Here's the drawing with two shaded views (mm, measured from the low corner). I have some questions. A direction names the side the tool comes from. Round coordinates to 2 decimals unless told otherwise and drop trailing zeros. Order: outer loops, then holes, each group sorted by start corner. A loop starts at its lowest first (then second) coordinate and runs counter-clockwise, first axis right, second up.
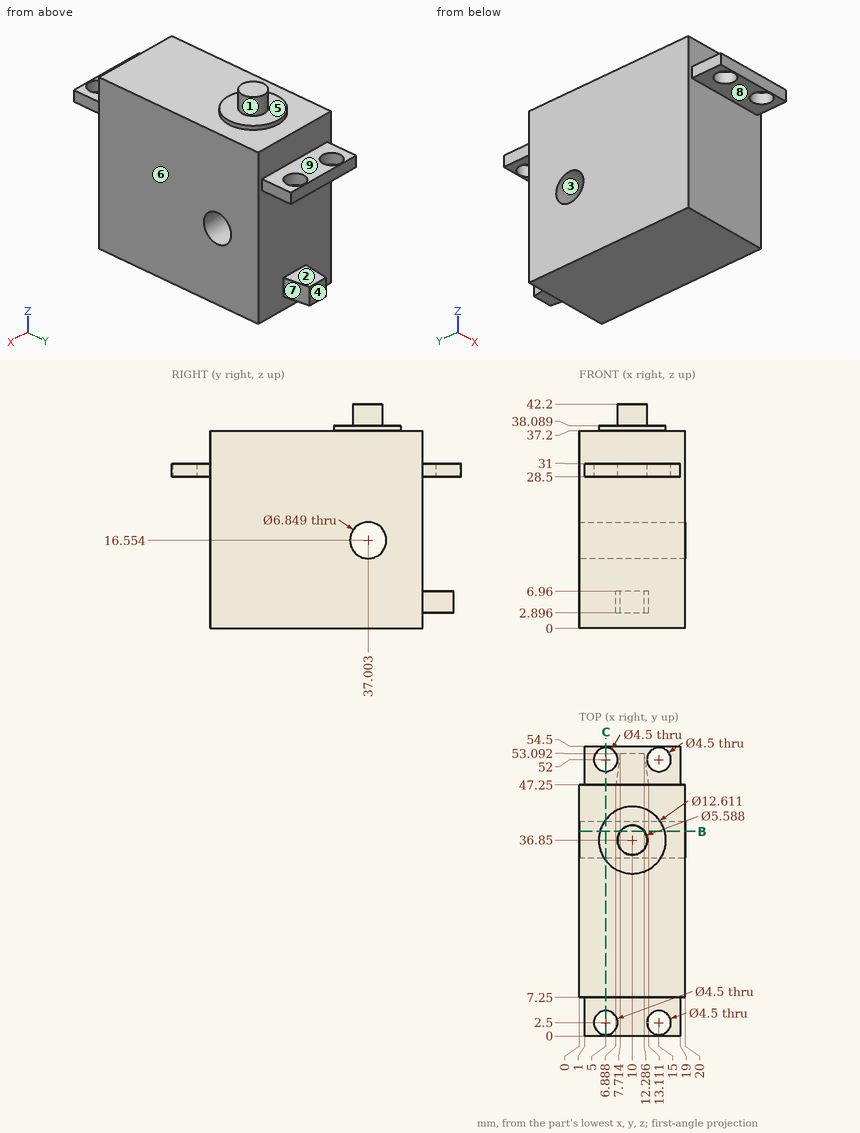
Q1. I need wall thicknesses on L1, parallel to Y at x = 5, z = 29; L2, parallel to Z at x = 16, y = 48.5; L3, parallel to Z at x = 15, y = 18.5. Which ranges of each line are inside material? Lowest first, please.
Q2. We'd pull the mould along Y, two halves only. Please class the marked faces 1, 2, 3 and 4: released by +Y, released by -Y, zero draft, split by the parting line, or undercut.
Q3. For P1, Ø1.5, axis at x = 6, z = 7, coming from the +Y side; P2, Ø6, axis at x = 5, y = 52, coming from the +Z side; P3, Ø6, axis at x = 14, z = 4, coming from the +Y side; P4, Ø5, axis at y = 28.5, z = 20, coming from the -X side, each with a flat end and sliding along its axis, tell me the tip position at first contact or that it passes through.
Q4. Imagine slicing it at B-B, the plane y = 38.5. Please give me the cut outline in (x, z) (1 decimal).
Q5. For the marked faces 5, 6, 7, 8 and 9, which set-ups out of +Z, -Z, +X, -X, +Y, -Y let a thin tool reach every point of the face, with its end or its side?
Q6. Imagine slicing it at C-C, the plane x = 5. State how many separate pieces and enclosed holes the cut face has, then the cut area to 3 significant figures.
Filled in:
1. L1: y = 0 to 0.25, 4.75 to 49.75, 54.25 to 54.5
1. L2: z = 28.5 to 31
1. L3: z = 0 to 37.2
2. face 1: split by the parting line
2. face 2: zero draft
2. face 3: undercut
2. face 4: released by +Y
3. P1: stops at y = 47.25
3. P2: stops at z = 31
3. P3: stops at y = 53.09
3. P4: stops at x = 0
4. outline: (0, 0) - (20, 0) - (20, 13.5) - (0, 13.5) - close; (0, 19.6) - (20, 19.6) - (20, 37.2) - (16.1, 37.2) - (16.1, 38.1) - (12.3, 38.1) - (12.3, 42.2) - (7.7, 42.2) - (7.7, 38.1) - (3.9, 38.1) - (3.9, 37.2) - (0, 37.2) - close
5. face 5: +Z
5. face 6: +Z, -Z, +X, +Y, -Y
5. face 7: -Z, +X, +Y
5. face 8: -Z, +X, -X, -Y
5. face 9: +Z, +X, -X, +Y
6. separate pieces: 3
6. enclosed holes: 1
6. area: 1,470 mm2
